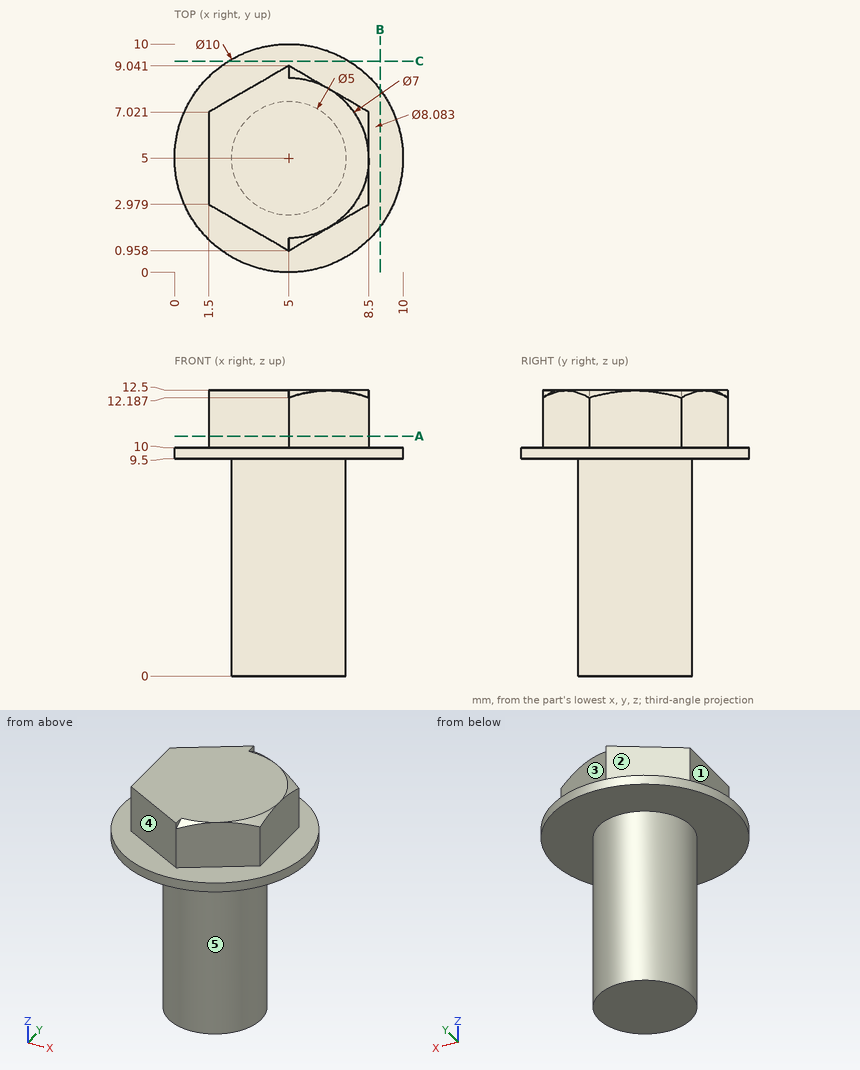
Can you work these out from the drawing? Everything is in mm from the part's minimum corner. A direction names the side the tool comes from. Give positions to 0.01 mm unless a question says otherwise; leave off trailing zeros. Loops run counter-clockwise (first coordinate to the right, second up) from the corner with the lowest first, then second, coordinate; pieces in that order, holes last. Notation, with made-up numbers: (15.5, 6.25) -> (64.5, 6.25) arc R29 ccw to (64.5, 39.25) -> close; hole circle Ø10 at (-19, 9.25). An arc over 180 degrees is marked (long way). Return JSON: item names as keys, results as strings.
Item 1: If we section it at C-C on y = 9.25: List the corners of the cut face in (x, z) for me.
Geometry results:
{"outline": "(2.37, 9.5) -> (7.63, 9.5) -> (7.63, 10) -> (2.37, 10) -> close"}
Item 2: I'm going to push a flat-ended pin straight in: pin 1 (1.2 mm diameter, centred on y = 4.5, z = 11, fed in from +X). Where does the tip first touch, or does it pass through?
Geometry results:
{"pin 1": "stops at x = 8.5"}
Item 3: If we section it at A-A on z = 10.5: List the corners of the cut face in (x, y) for me.
Geometry results:
{"outline": "(1.5, 2.98) -> (5, 0.96) -> (8.5, 2.98) -> (8.5, 7.02) -> (5, 9.04) -> (1.5, 7.02) -> close"}
Item 4: Which directions (+Z, -Z, +X, -X, +Y, -Y) give clear straight access to the entire face, cutting with the end or side of a thin tool? Please do the marked faces 1, 2, 3, 4 and 5.
Geometry results:
{"face 1": "+Z, -X, +Y, -Y", "face 2": "+Z, -X, +Y", "face 3": "+Z, +X, +Y", "face 4": "+Z, -X, -Y", "face 5": "-Z"}
Item 5: I need wall thicknesses on L1, parallel to Z at x = 5.25, y = 1.75; L2, parallel to X at y = 3, z = 10.5; L3, parallel to Z at x = 2, y = 7.5. Which ranges of each line are inside material? Lowest first, please. Write a range as from..to.
Geometry results:
{"L1": "z = 9.5..12.5", "L2": "x = 1.5..8.5", "L3": "z = 9.5..10"}
Item 6: If we section it at B-B on x = 9: List the corners of the cut face in (y, z) for me.
Geometry results:
{"outline": "(2, 9.5) -> (8, 9.5) -> (8, 10) -> (2, 10) -> close"}
